The listing builds one solid part. Answer for the finished solid, in the listing's coordinates (mm). Round coordinates to 2 decimals unless told otherwise and drop trailing zeros. Write each loop counter-clockwise with the first axis right and the second up, starting at its lowest first coordinate (ties: lowest second). Pieces come first, ordered by that corner, then holes. Notation, with made-up numbers: M -16.5,-7 L 33.5,-7 A21 ccw 33.5,0 Z; hole C 30.25,24.5 d10. An arc over 180 degrees is marked long. Answer as CSV lines item,"result". Start each with the question number.
from build123d import *

# Parameters (mm, degrees)
F0_R     = 50
F1_DEPTH = 10
F2_R     = 125
F2_R_2   = 40.44952
F3_DEPTH = 10
F5_DEPTH = 25
F6_R     = 97.834201
F7_DEPTH = 25


with BuildPart() as f1:
    # F0 (on Top) → F1 (new body)
    with BuildSketch(Plane.XY):
        Circle(F0_R)
        Polygon((-10, 30), (0, 30), (10, 30), (10, 10), (30, 10), (30, 0), (30, -10), (10, -10), (10, -30), (0, -30), (-10, -30), (-10, -10), (-30, -10), (-30, 0), (-30, 10), (-10, 10), align=None, mode=Mode.SUBTRACT)
    extrude(amount=F1_DEPTH)

    # F2 (on face) → F3 (join)
    with BuildSketch(Plane.XY.offset(10)):
        Circle(F2_R)
        Circle(F2_R_2, mode=Mode.SUBTRACT)
    extrude(amount=-F3_DEPTH)

    # F4 (on face) → F5 (cut)
    with BuildSketch(Plane.XY.offset(10)):
        with BuildLine():
            Line((0, 116.456337), (0, 104.802647))
            ThreePointArc((0, 104.802647), (9.134153, 104.403842), (18.198789, 103.21046))
            Line((18.198789, 103.21046), (20.222431, 114.687104))
            ThreePointArc((20.222431, 114.687104), (10.149839, 116.013186), (0, 116.456337))
        make_face()
        with BuildLine():
            ThreePointArc((-35.844616, 98.482274), (-27.124921, 101.231584), (-18.198789, 103.21046))
            Line((-18.198789, 103.21046), (-20.222431, 114.687104))
            ThreePointArc((-20.222431, 114.687104), (-30.141118, 112.488184), (-39.830413, 109.433161))
            Line((-39.830413, 109.433161), (-35.844616, 98.482274))
        make_face()
        with BuildLine():
            ThreePointArc((-67.365843, 80.283486), (-60.112329, 85.849303), (-52.401324, 90.761755))
            Line((-52.401324, 90.761755), (-58.228169, 100.854147))
            ThreePointArc((-58.228169, 100.854147), (-66.796611, 95.395447), (-74.856691, 89.21073))
            Line((-74.856691, 89.21073), (-67.365843, 80.283486))
        make_face()
        with BuildLine():
            ThreePointArc((-90.761755, 52.401324), (-85.849303, 60.112329), (-80.283486, 67.365843))
            Line((-80.283486, 67.365843), (-89.21073, 74.856691))
            ThreePointArc((-89.21073, 74.856691), (-95.395447, 66.796611), (-100.854147, 58.228169))
            Line((-100.854147, 58.228169), (-90.761755, 52.401324))
        make_face()
        with BuildLine():
            ThreePointArc((-103.21046, 18.198789), (-101.231584, 27.124921), (-98.482274, 35.844616))
            Line((-98.482274, 35.844616), (-109.433161, 39.830413))
            ThreePointArc((-109.433161, 39.830413), (-112.488184, 30.141118), (-114.687104, 20.222431))
            Line((-114.687104, 20.222431), (-103.21046, 18.198789))
        make_face()
        with BuildLine():
            ThreePointArc((-103.21046, -18.198789), (-104.403842, -9.134153), (-104.802647, 0))
            Line((-104.802647, 0), (-116.456337, 0))
            ThreePointArc((-116.456337, 0), (-116.013186, -10.149839), (-114.687104, -20.222431))
            Line((-114.687104, -20.222431), (-103.21046, -18.198789))
        make_face()
        with BuildLine():
            ThreePointArc((-90.761755, -52.401324), (-94.983455, -44.291513), (-98.482274, -35.844616))
            Line((-98.482274, -35.844616), (-109.433161, -39.830413))
            ThreePointArc((-109.433161, -39.830413), (-105.545285, -49.216575), (-100.854147, -58.228169))
            Line((-100.854147, -58.228169), (-90.761755, -52.401324))
        make_face()
        with BuildLine():
            ThreePointArc((-67.365843, -80.283486), (-74.106663, -74.106663), (-80.283486, -67.365843))
            Line((-80.283486, -67.365843), (-89.21073, -74.856691))
            ThreePointArc((-89.21073, -74.856691), (-82.347066, -82.347066), (-74.856691, -89.21073))
            Line((-74.856691, -89.21073), (-67.365843, -80.283486))
        make_face()
        with BuildLine():
            ThreePointArc((-35.844616, -98.482274), (-44.291513, -94.983455), (-52.401324, -90.761755))
            Line((-52.401324, -90.761755), (-58.228169, -100.854147))
            ThreePointArc((-58.228169, -100.854147), (-49.216575, -105.545285), (-39.830413, -109.433161))
            Line((-39.830413, -109.433161), (-35.844616, -98.482274))
        make_face()
        with BuildLine():
            ThreePointArc((0, -104.802647), (-9.134153, -104.403842), (-18.198789, -103.21046))
            Line((-18.198789, -103.21046), (-20.222431, -114.687104))
            ThreePointArc((-20.222431, -114.687104), (-10.149839, -116.013186), (0, -116.456337))
            Line((0, -116.456337), (0, -104.802647))
        make_face()
        with BuildLine():
            ThreePointArc((35.844616, -98.482274), (27.124921, -101.231584), (18.198789, -103.21046))
            Line((18.198789, -103.21046), (20.222431, -114.687104))
            ThreePointArc((20.222431, -114.687104), (30.141118, -112.488184), (39.830413, -109.433161))
            Line((39.830413, -109.433161), (35.844616, -98.482274))
        make_face()
        with BuildLine():
            ThreePointArc((67.365843, -80.283486), (60.112329, -85.849303), (52.401324, -90.761755))
            Line((52.401324, -90.761755), (58.228169, -100.854147))
            ThreePointArc((58.228169, -100.854147), (66.796611, -95.395447), (74.856691, -89.21073))
            Line((74.856691, -89.21073), (67.365843, -80.283486))
        make_face()
        with BuildLine():
            ThreePointArc((90.761755, -52.401324), (85.849303, -60.112329), (80.283486, -67.365843))
            Line((80.283486, -67.365843), (89.21073, -74.856691))
            ThreePointArc((89.21073, -74.856691), (95.395447, -66.796611), (100.854147, -58.228169))
            Line((100.854147, -58.228169), (90.761755, -52.401324))
        make_face()
        with BuildLine():
            ThreePointArc((103.21046, -18.198789), (101.231584, -27.124921), (98.482274, -35.844616))
            Line((98.482274, -35.844616), (109.433161, -39.830413))
            ThreePointArc((109.433161, -39.830413), (112.488184, -30.141118), (114.687104, -20.222431))
            Line((114.687104, -20.222431), (103.21046, -18.198789))
        make_face()
        with BuildLine():
            ThreePointArc((103.21046, 18.198789), (104.403842, 9.134153), (104.802647, 0))
            Line((104.802647, 0), (116.456337, 0))
            ThreePointArc((116.456337, 0), (116.013186, 10.149839), (114.687104, 20.222431))
            Line((114.687104, 20.222431), (103.21046, 18.198789))
        make_face()
        with BuildLine():
            ThreePointArc((90.761755, 52.401324), (94.983455, 44.291513), (98.482274, 35.844616))
            Line((98.482274, 35.844616), (109.433161, 39.830413))
            ThreePointArc((109.433161, 39.830413), (105.545285, 49.216575), (100.854147, 58.228169))
            Line((100.854147, 58.228169), (90.761755, 52.401324))
        make_face()
        with BuildLine():
            ThreePointArc((67.365843, 80.283486), (74.106663, 74.106663), (80.283486, 67.365843))
            Line((80.283486, 67.365843), (89.21073, 74.856691))
            ThreePointArc((89.21073, 74.856691), (82.347066, 82.347066), (74.856691, 89.21073))
            Line((74.856691, 89.21073), (67.365843, 80.283486))
        make_face()
        with BuildLine():
            ThreePointArc((35.844616, 98.482274), (44.291513, 94.983455), (52.401324, 90.761755))
            Line((52.401324, 90.761755), (58.228169, 100.854147))
            ThreePointArc((58.228169, 100.854147), (49.216575, 105.545285), (39.830413, 109.433161))
            Line((39.830413, 109.433161), (35.844616, 98.482274))
        make_face()
    extrude(amount=-F5_DEPTH, mode=Mode.SUBTRACT)

    # F6 (on face) → F7 (cut)
    with BuildSketch(Plane.XY.offset(10)):
        Circle(F6_R)
    extrude(amount=-F7_DEPTH, mode=Mode.SUBTRACT)


solid = f1.part
Q1. Find section C-C (x = 71.5). Determine the outline of the cut face in (y, z), plus the area to 3 significant figures.
Q2. Find section B-B (x = -45). Determine the outline of the cut face in (y, z).
Q3. Find section A-A (y = -14). Determine the outline of the cut face in (x, z), plus the area to 3 significant figures.
Q4. Straight lines are drawn through the part: L1, parallel to X at y = 91, z = 4.5; L2, parallel to Y at x = 42.5, z = 2.5; L3, parallel to X at y = -83, z = 2.5. For each, find the intervals that lie inside material, in ascending order.
Q5. Find section D-D (z = 7.5). Count the separate pieces of the cut face and the enclosed holes in it, plus the area to 3 significant figures.
Q6. Each of these flat-tipped pins is pushed along its axis until it touches: P1, Ø3, axis at y = 112.5, z = 6, coming from the +X side; P2, Ø6, axis at x = -13, z = 5, coming from the +Y side; P3, Ø3, axis at x = 112, z = 6, coming from the +Y side. Where does it stop, or does it pass through?
Reported:
1,outline,"M -102.53,0 L -91.92,0 L -91.92,10 L -102.53,10 Z; M -85.21,0 L -66.78,0 L -66.78,10 L -85.21,10 Z; M 66.78,0 L 76.62,0 L 76.62,10 L 66.78,10 Z; M 85.21,0 L 102.53,0 L 102.53,10 L 85.21,10 Z"
1,area,"562 mm2"
2,outline,"M -116.62,0 L -107.41,0 L -107.41,10 L -116.62,10 Z; M -94.65,0 L -86.87,0 L -86.87,10 L -94.65,10 Z; M 86.87,0 L 116.62,0 L 116.62,10 L 86.87,10 Z"
3,outline,"M -124.21,0 L -115.61,0 L -115.61,10 L -124.21,10 Z; M -103.86,0 L -96.83,0 L -96.83,10 L -103.86,10 Z; M 96.83,0 L 124.21,0 L 124.21,10 L 96.83,10 Z"
3,area,"430 mm2"
4,L1,"x = -85.7 to -72.67, -52.54 to -35.92, 35.92 to 51.99, 52.54 to 85.7"
4,L2,"y = -117.55 to -88.12, 88.12 to 95.8, 108.42 to 117.55"
4,L3,"x = -93.47 to -81.69, -69.65 to -51.79, 51.79 to 63.99, 69.65 to 93.47"
5,separate pieces,"1"
5,enclosed holes,"19"
5,area,"15,000 mm2"
6,P1,"stops at x = 57.48"
6,P2,"stops at y = 124.6"
6,P3,"stops at y = 58.44"
